from build123d import *

# Parameters (mm, degrees)
SKETCH1_R           = 1.5
BOSS_EXTRUDE1_DEPTH = 3
BOSS_EXTRUDE2_DEPTH = 25.2
SKETCH6_W           = 57.536590271
SKETCH6_H           = 9.11547301
CUT_EXTRUDE1_DEPTH  = 64.271846515
FILLET1_R           = 2
FILLET2_R           = 1


with BuildPart() as part:
    # Sketch1 → Boss-Extrude1 (new body)
    with BuildSketch(Plane.XY):
        with BuildLine():
            Line((3.68220241, -19.5), (18.54616344, -19.5))
            ThreePointArc((18.54616344, -19.5), (19.008103207, -19.191341716), (18.899716831, -18.646446609))
            Line((18.899716831, -18.646446609), (3.854153503, -3.600883281))
            ThreePointArc((3.854153503, -3.600883281), (3.30197574, -2.551779506), (3.440748076, -1.374383543))
            ThreePointArc((3.440748076, -1.374383543), (2.199066013, 3.02009221), (-2.348238623, 2.601508845))
            Line((-2.348238623, 2.601508845), (-4.469558967, 0.480188501))
            ThreePointArc((-4.469558967, 0.480188501), (-5.055345405, -0.934025061), (-4.469558967, -2.348238623))
            Line((-4.469558967, -2.348238623), (1.803522753, -8.621320344))
            ThreePointArc((1.803522753, -8.621320344), (2.453841007, -9.59459039), (2.68220241, -10.742640687))
            Line((2.68220241, -10.742640687), (2.68220241, -18.5))
            ThreePointArc((2.68220241, -18.5), (2.975095629, -19.207106781), (3.68220241, -19.5))
        make_face()
        Circle(SKETCH1_R, mode=Mode.SUBTRACT)
    boss_extrude1 = extrude(amount=BOSS_EXTRUDE1_DEPTH)

    # Sketch2 → Boss-Extrude2 (add)
    with BuildSketch(Plane.XY.offset(3)):
        with BuildLine():
            Line((18.899716831, -18.646446609), (10.995910909, -10.742640687))
            Line((10.995910909, -10.742640687), (2.68220241, -10.742640687))
            Line((2.68220241, -10.742640687), (2.68220241, -18.5))
            ThreePointArc((2.68220241, -18.5), (2.975095629, -19.207106781), (3.68220241, -19.5))
            Line((3.68220241, -19.5), (18.54616344, -19.5))
            ThreePointArc((18.54616344, -19.5), (19.008103207, -19.191341716), (18.899716831, -18.646446609))
        make_face()
    boss_extrude2 = extrude(amount=BOSS_EXTRUDE2_DEPTH)

    # Mirror1: Boss-Extrude1, Boss-Extrude2 across plane
    add(boss_extrude1.mirror(Plane.XY.offset(28.2)))
    add(boss_extrude2.mirror(Plane.XY.offset(28.2)))

    # Sketch6 → Cut-Extrude1 (cut, through all)
    with BuildSketch(Plane(origin=(-6.530219139, -6.530219139, 0), x_dir=(0, 0, 1), z_dir=(-0.7071067811865487, -0.7071067811865465, 0))):
        with Locations((27.631704865, -17.586068001)):
            Rectangle(SKETCH6_W, SKETCH6_H)
    extrude(amount=CUT_EXTRUDE1_DEPTH, mode=Mode.SUBTRACT)

    # Fillet1
    fillet1_edges = [part.edges().sort_by_distance(p)[0] for p in [
        (6.439561723, -19.5, 28.2),
    ]]
    fillet(fillet1_edges, radius=FILLET1_R)

    # Fillet2
    fillet2_edges = [part.edges().sort_by_distance(p)[0] for p in [
        (2.68220241, -15.742640687, 28.2),
    ]]
    fillet(fillet2_edges, radius=FILLET2_R)


solid = part.part
Could you check a few things on this model? Use its own coordinates, in mm. A direction names the side the tool comes from. Give positions to 0.01 mm unless a question says otherwise; leave off trailing zeros. Write each loop counter-clockwise with the first axis right and the second up, starting at its lowest first coordinate (ties: lowest second). Pieces come first, ordered by that corner, then holes. Notation, with made-up numbers: (-17.5, 21) - (15.5, 21) arc R32 ccw to (15.5, 48) - close; hole circle Ø3 at (-2.5, 48). An arc over 180 degrees is marked (long way). Use CSV: the item, a comma, the result in double quotes. Start each with the question number.
Item 1: I'm going to push flat-ended pins straight in: pin 1 (1 mm diameter, centred on x = 14.5, z = 9, fed in from +Y); pin 2 (2.5 mm diameter, centred on y = -13.5, z = 30.5, fed in from -X); pin 3 (4 mm diameter, centred on x = 5.5, z = 25.5, fed in from +Y). Where does each tip first touch, or does it pass through?
Item 2: If we mould it in two halves opening along Y, with no side actions, what happens to faces 1 (the face through (-5.055, -0.912, 1.479)), 2 (the face through (7, -10.743, 29)), 3 (the face through (-1.5, 0.07, 1.48)), 4 (the face through (3.305, -2.568, 1.479))? For each: pulls with the +Y half, pulls with the -Y half, needs draft (parallel to the pull), parting line crosses it, or undercut.
Item 3: I want a section at C-C, the plane z = 32. Please give me the cut outline in (x, y), then the cut area to 3 significant figures.
Item 4: I want a section at A-A, the plane x = -3.25. Please give me the cut outline in (y, z), then the cut area to 3 significant figures.
Item 5: For faces 5 (the face through (3, -3, 53.4)), 6 (the face through (2.447, -9.579, 54.921)), which set-ups out of +Z, -Z, +X, -X, +Y, -Y let a thin tool reach every point of the face, with its end or its side?
Item 6: I want a section at B-B, the plane y = -3. Please give me the cut outline in (x, z), then the cut area to 3 significant figures.
Item 7: If I drill on line 1 along Z through (x, y) = (6.5, -7.75); line 2 along Y through (x, z) = (0, 55.3); line 3 along Y through (x, z) = (4.5, 43.5), over which ranges is the centre line in solid material (lowest first)?
Item 8: I want a section at D-D, the plane x = 0. Please give me the cut outline in (y, z), then the cut area to 3 significant figures.
Findings:
1,pin 1,"stops at y = -13.75"
1,pin 2,"stops at x = 2.68"
1,pin 3,"stops at y = -10.74"
2,face 1,"parting line crosses it"
2,face 2,"pulls with the +Y half"
2,face 3,"undercut"
2,face 4,"undercut"
3,outline,"(2.68, -15.33) arc R1 ccw to (2.98, -16.04) - (5.85, -18.91) arc R2 ccw to (7.27, -19.5) - (18.55, -19.5) arc R0.5 ccw to (18.9, -18.65) - (11, -10.74) - (2.68, -10.74) - close"
3,area,"104 mm2"
4,outline,"(-3.57, 0) - (1.7, 0) - (1.7, 3) - (-3.57, 3) - close; (-3.57, 53.4) - (1.7, 53.4) - (1.7, 56.4) - (-3.57, 56.4) - close"
4,area,"31.6 mm2"
5,face 5,"+X, -X, +Y"
5,face 6,"+Z, -Z, -X, -Y"
6,outline,"(-3.82, 0) - (3.44, 0) - (3.44, 3) - (-3.82, 3) - close; (-3.82, 53.4) - (3.44, 53.4) - (3.44, 56.4) - (-3.82, 56.4) - close"
6,area,"43.6 mm2"
7,line 1,"z = 0 to 3, 53.4 to 56.4"
7,line 2,"y = -6.82 to -1.5, 1.5 to 3.64"
7,line 3,"y = -17.56 to -10.74"
8,outline,"(-6.82, 0) - (-1.5, 0) - (-1.5, 3) - (-6.82, 3) - close; (-6.82, 53.4) - (-1.5, 53.4) - (-1.5, 56.4) - (-6.82, 56.4) - close; (1.5, 0) - (3.64, 0) - (3.64, 3) - (1.5, 3) - close; (1.5, 53.4) - (3.64, 53.4) - (3.64, 56.4) - (1.5, 56.4) - close"
8,area,"44.8 mm2"
